For this review, use the dimensioned drawing (mm, ordinates from the lowest corner) and the shaded views. A direction names the side the tool comes from. Round coordinates to 2 decimals unless told otherwise and drop trailing zeros. Write each loop counter-clockwise with the first axis right and the second up, starting at its lowest first coordinate (ties: lowest second). Pieces come first, ordered by that corner, then holes. Notation, with made-up numbers: M 6.25,-10.5 L 18.25,-10.5 A12 ccw 18.25,1.5 Z; hole C 12,-18.75 d7. An arc over 180 degrees is marked long. Use CSV: the item, a comma, the result in double quotes.
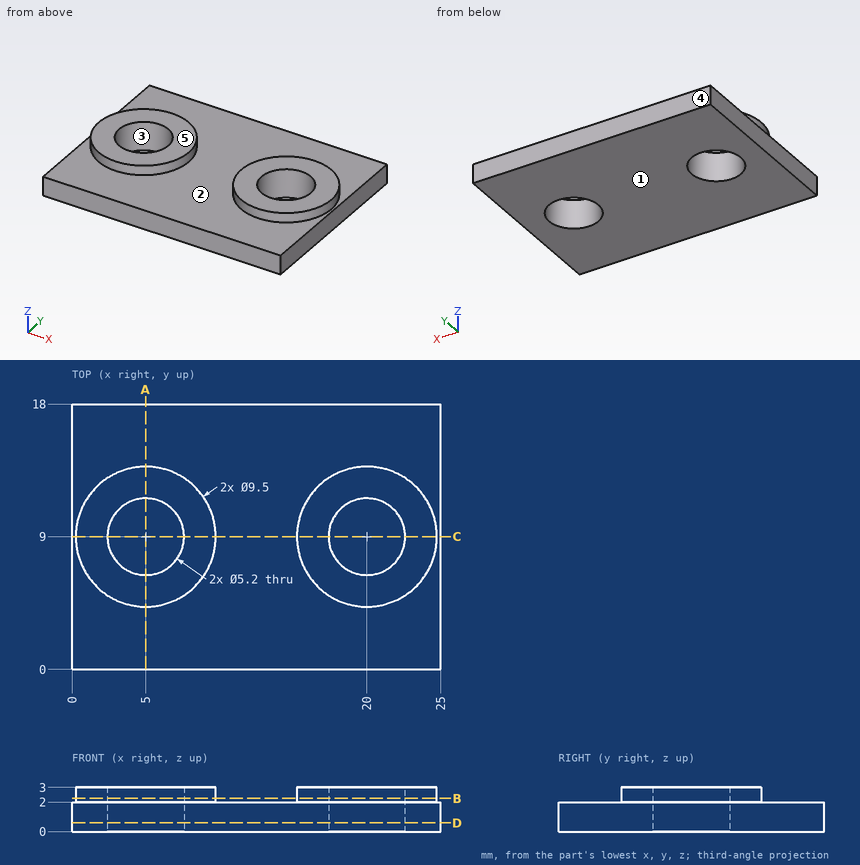
1) Add section D-D on z = 0.6. Write out the cut boundary in (x, y), then the cut area to 3 significant figures.
Answers:
outline,"M 0,0 L 25,0 L 25,18 L 0,18 Z; hole C 5,9 d5.2; hole C 20,9 d5.2"
area,"408 mm²"
2) Add section A-A on x = 5. Write out the cut boundary in (y, z).
Answers:
outline,"M 0,0 L 6.4,0 L 6.4,3 L 4.25,3 L 4.25,2 L 0,2 Z; M 11.6,0 L 18,0 L 18,2 L 13.75,2 L 13.75,3 L 11.6,3 Z"
3) Wall thickness on line 1 along Y through (x, z) = (5, 0.95); line 2 along Y through (x, z) = (5, 2.35); line 3 along Z through (x, y) = (11, 4.75): over which ranges is each line inside the solid? List them lowest first. Write a range as [from, to].
Answers:
line 1,"[0, 6.4], [11.6, 18]"
line 2,"[4.25, 6.4], [11.6, 13.75]"
line 3,"[0, 2]"
4) The part is to be moulded in two halves that separate along Y. For the marked faces 3, 4 and 5, say which applies: released by +Y, released by -Y, zero draft, split by the parting line, or undercut.
Answers:
face 3,"undercut"
face 4,"released by +Y"
face 5,"zero draft"
5) Add section C-C on y = 9. Write out the cut boundary in (x, z).
Answers:
outline,"M 0,0 L 2.4,0 L 2.4,3 L 0.25,3 L 0.25,2 L 0,2 Z; M 7.6,0 L 17.4,0 L 17.4,3 L 15.25,3 L 15.25,2 L 9.75,2 L 9.75,3 L 7.6,3 Z; M 22.6,0 L 25,0 L 25,2 L 24.75,2 L 24.75,3 L 22.6,3 Z"
6) Add section B-B on z = 2.25. Write out the cut boundary in (x, y).
Answers:
outline,"C 5,9 d9.5; C 20,9 d9.5; hole C 5,9 d5.2; hole C 20,9 d5.2"
7) Machinability: for the marked faces 1 and 2, which of the approach directions +Z, -Z, +X, -X, +Y, -Y give a long, thin tool a straight path to every point of the face, cutting with its end or side? Answer none if there is none.
Answers:
face 1,"-Z, +X, -X, +Y, -Y"
face 2,"+Z"
8) For pin 1 Ø1.5 at (x, y) = (15.5, 12.5) entering from +Z, flat-tipped, find the tip position at first contact; note if it passes through.
Answers:
pin 1,"z = 2"
